Work out the finished part from the listing and answer in its coordinate system (mm). Face numbers are marked on the shaded views. A direction names the side the tool comes from. Coordinates: 2 decimals unless noted, no trailing zeros. Order: outer loops, then holes, each group sorted by start corner. A loop starts at its lowest first (then second) coordinate and runs counter-clockwise, first axis right, second up. Notation, with made-up numbers: (2.25, 76) -> (59.25, 76) arc R15 ccw to (59.25, 92) -> close; hole circle Ø10 at (52, 75.5). An arc over 180 degrees is marked (long way). Use one line per item in the form item = value.
from build123d import *

# Parameters (mm, degrees)
F0_R     = 13.7004804212
F1_DEPTH = 25
F2_COUNT = 12


with BuildPart() as f1:
    # F0 (on Front) → F1 (new body)
    with BuildSketch(Plane.XZ):
        with BuildLine():
            ThreePointArc((5.1877617459, 15.4656955182), (1.3348337551, 15.7425763881), (-2.5179670171, 15.4639308632))
            ThreePointArc((-2.5179670171, 15.4639308632), (-5.3039752447, 14.9076599703), (-8.0156462094, 14.0602405167))
            ThreePointArc((-8.0156462094, 14.0602405167), (-10.1642311279, 13.1537985607), (-12.2260978725, 12.064413551))
            ThreePointArc((-12.2260978725, 12.064413551), (-14.7363892101, 10.3996164513), (-17.044498214, 8.4642237758))
            ThreePointArc((-17.044498214, 8.4642237758), (-19.1213988999, 6.2825744141), (-20.9409732492, 3.8821037136))
            ThreePointArc((-20.9409732492, 3.8821037136), (-22.4803390837, 1.292998939), (-23.7201379517, -1.4521803764))
            ThreePointArc((-23.7201379517, -1.4521803764), (-24.6447786512, -4.3189119634), (-25.2426333118, -7.2711450539))
            ThreePointArc((-25.2426333118, -7.2711450539), (-25.5061835733, -10.2717538785), (-25.4321150685, -13.2830037711))
            ThreePointArc((-25.4321150685, -13.2830037711), (-25.0213593458, -16.2670260316), (-24.2790819112, -19.1862953452))
            ThreePointArc((-24.2790819112, -19.1862953452), (-23.2146169595, -22.0041010545), (-21.8413509371, -24.6850067))
            ThreePointArc((-21.8413509371, -24.6850067), (-20.1765542068, -27.195297335), (-18.2411620449, -29.5034057391))
            ThreePointArc((-18.2411620449, -29.5034057391), (-16.0595125704, -31.5803065899), (-13.6590417261, -33.3998810729))
            ThreePointArc((-13.6590417261, -33.3998810729), (-11.0699368198, -34.9392469858), (-8.3247573578, -36.1790459013))
            ThreePointArc((-8.3247573578, -36.1790459013), (-5.4580256945, -37.1036865942), (-2.5057925274, -37.701541232))
            ThreePointArc((-2.5057925274, -37.701541232), (0.494815816, -37.9650914367), (3.5060652253, -37.8910229838))
            ThreePointArc((3.5060652253, -37.8910229838), (6.490087912, -37.4802672463), (9.4093576356, -36.7379897032))
            ThreePointArc((9.4093576356, -36.7379897032), (12.2271632206, -35.6735247759), (14.9080687518, -34.3002588042))
            ThreePointArc((14.9080687518, -34.3002588042), (17.418359676, -32.6354618578), (19.7264683173, -30.7000694179))
            ThreePointArc((19.7264683173, -30.7000694179), (21.8033689519, -28.5184200728), (23.6229432563, -26.1179493978))
            ThreePointArc((23.6229432563, -26.1179493978), (25.1623091778, -23.5288444178), (26.4021080868, -20.7836648785))
            ThreePointArc((26.4021080868, -20.7836648785), (27.3267486462, -17.9169335612), (27.9246032308, -14.9647007613))
            ThreePointArc((27.9246032308, -14.9647007613), (28.132175105, -13.0462877166), (28.2014849595, -11.1179229076))
            ThreePointArc((28.2014849595, -11.1179229076), (28.1796260721, -10.0345007945), (28.1140849874, -8.9528420441))
            ThreePointArc((28.1140849874, -8.9528420441), (27.7033292139, -5.9688195233), (26.9610516709, -3.0495499642))
            ThreePointArc((26.9610516709, -3.0495499642), (25.8965868926, -0.2317447927), (24.5233211592, 2.4491603668))
            ThreePointArc((24.5233211592, 2.4491603668), (22.8585242407, 4.9594513659), (20.923131816, 7.2675600815))
            ThreePointArc((20.923131816, 7.2675600815), (18.7414824625, 9.3444607976), (16.3410117658, 11.1640351765))
            ThreePointArc((16.3410117658, 11.1640351765), (13.7519066478, 12.703401218), (11.0067269497, 13.9432002123))
            ThreePointArc((11.0067269497, 13.9432002123), (8.1399951015, 14.867840913), (5.1877617459, 15.4656955182))
        make_face()
        with Locations((1.3409849595, -11.1179229076)):
            Circle(F0_R, mode=Mode.SUBTRACT)
        with BuildLine():
            ThreePointArc((-8.0156462094, 14.0602405167), (-5.3039752447, 14.9076599703), (-2.5179670171, 15.4639308632))
            ThreePointArc((-2.5179670171, 15.4639308632), (-2.7094878329, 19.7420226798), (-4.1807882522, 23.7637169608))
            Line((-4.1807882522, 23.7637169608), (-5.1883789909, 24.5569822892))
            Line((-5.1883789909, 24.5569822892), (-7.8406668751, 22.2773347298))
            ThreePointArc((-7.8406668751, 22.2773347298), (-8.4992599438, 18.1809490139), (-8.0156462094, 14.0602405167))
        make_face()
    extrude(amount=F1_DEPTH)

    # F2: F1 ×12 about axis
    f2_axis = Axis((1.3409849595, 0, -11.1179229076), (0, 1, 0))


with BuildPart() as f1_1:
    add(f1.part)
    for i in range(1, F2_COUNT):
        add(f1.part.rotate(f2_axis, i * 360 / F2_COUNT))


solid = f1_1.part
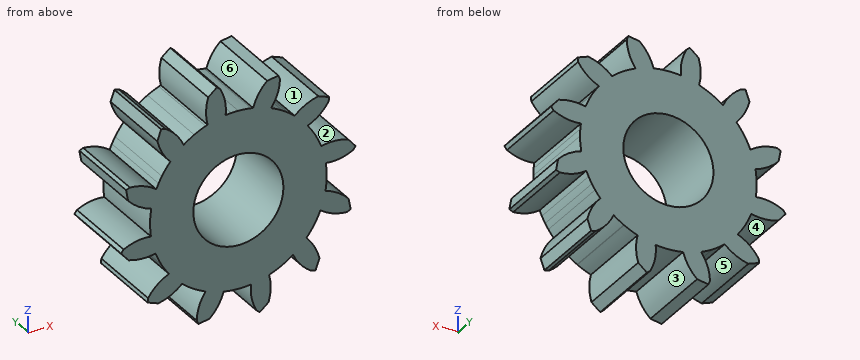
(1) Each of these flat-tipped pins is pushed along its axis until it touches: P1, Ø5, axis at y = -10.5, z = -12, coming from the +X side; P2, Ø12, axis at x = 23, y = -4.5, coming from the -Z side; P3, Ø4, axis at x = -13.5, y = -15.5, coming from the +Z side. Where does it stop, or does it pass through?
Data:
P1 = 28.2
P2 = -38.75
P3 = 12.47
(2) Which of the six approach directions +Z, -Z, +X, -X, +Y, -Y give full straight-line access (tool end or side, diameter ignored) to the marked faces 4, 5 and 6?
Data:
face_4 = +Y, -Y
face_5 = -Z, +Y, -Y
face_6 = +Z, +Y, -Y
(3) Straight lines are drawn through the part: line 1 along Z through (x, y) = (13, -5.75); line 2 along Z through (x, y) = (12, -18.75); line 3 along X through (y, z) = (-11, -1). For each, find the intervals that lie inside material, in ascending order.
Data:
line_1 = -35.32 to -18.31, -3.92 to 13.08, 16.92 to 22.94
line_2 = -35.77 to -19.73, -2.51 to 13.54, 14.9 to 22.75
line_3 = -32.43 to -23.84, -23.54 to -7.9, 10.58 to 26.22
(4) Section A-A on x = -28 is taken. Write down the section's boundary in (y, z).
Data:
outline = (-25, -20.96) -> (0, -20.96) -> (0, -14.95) -> (-25, -14.95) -> close; (-25, -5.52) -> (0, -5.52) -> (0, 0.99) -> (-25, 0.99) -> close
(5) Section B-B on z = -18.5 is taken. Write down the section's boundary in (x, y), plus the area to 3 significant figures.
Data:
outline = (-33.6, -25) -> (-10.2, -25) -> (-10.2, 0) -> (-33.6, 0) -> close; (12.88, -25) -> (33.4, -25) -> (33.4, 0) -> (12.88, 0) -> close
area = 1,100 mm²
(6) The mould has two halves that part along Z. Classify the marked faces 1, 2 and 3: released by +Z, released by -Z, zero draft, split by the parting line, or undercut.
Data:
face_1 = released by +Z
face_2 = undercut
face_3 = released by -Z
